The model under review builds one solid part; all positions refer to its coordinate system, in mm. A direction names the side the tool comes from. Coordinates: 2 decimals unless noted, no trailing zeros. Write each loop counter-clockwise with the first axis right and the second up, starting at its lowest first coordinate (ties: lowest second). Pieces come first, ordered by that corner, then holes.
1) Add section A-A, the plane z = -8.5. State the section outline as (x, y) points.
2) Machinability: for faces 1 (the flat face through (-1.65, -1.74, 3.77)), 2 (the cylindrical face through (-0.54, 2.44, -10.31)), which of the approach directions +Z, -Z, +X, -X, +Y, -Y give a long, thin tool a straight path to every point of the face, cutting with its end or side? Answer none if there is none.
3) For P1, Ø1, axis at y = -1, z = -2.5, coming from the -X side; P2, Ø1, axis at x = 1, y = 3.5, coming from the -Z side; P3, Ø0.9, axis at x = 1, y = -1.5, coming from the +Z side, all flat-tipped, find the tip position at first contact; note any pin that passes through.
4) For line 1 (Z direction, x = 3, y = -1); line 2 (Y direction, x = 0, z = -1.75); line 3 (X direction, y = 1.5, z = -19), list the stretches that pass through material, from the lowest coordinate up.
5) Mouldability with a two-part tool opening along X and no side actions: class faces 3 (the cylindrical face through (2.285, -3.584, 2.469)), 4 (the flat face through (1.65, 1.74, 3.77)), 5 (the flat face through (2, -2, 5)) as released by +X, released by -X, zero draft, split by the parting line, or undercut.
Solid Edge part; units mm, degrees
sketch "Sketch1" plane through (0, 0, 0) normal (0, -1, 0) x (1, 0, 0)
  line L0 (4.25, 5) -> (4.25, 0)
  line L1 (4.25, 0) -> (2.85, 0)
  line L2 (2.85, 0) -> (2.5, -0.6062)
  line L3 (2.5, -0.6062) -> (2.5, -20)
  line L4 (2.5, -20) -> (0, -20)
  line L5 (2.3, 2.5) -> (0, 1.1721)
  line L6 (2.3, 5) -> (2.3, 2.5)
  line L7 (4.25, 5) -> (2.3, 5)
revolve "RevolvedProtrusion1" add sketch "Sketch1" angle 360 about axis through (0, 0, -6) along (0, 0, 1)
cosmetic_thread "Thread1"
chamfer "Chamfer_1" distance 0.25 angle 45 1 edges at (-2.5, 0, -20)
fillet "Round_1" radius 0.3 2 edges at (-4.25, 0, 0) (-4.25, 0, 5)
sketch "Sketch2" plane through (0, 0, 5) normal (0, 0, 1) x (0, 1, 0)
  line L0 (-2.3, 1.3279) -> (-2.3, -1.3279)
  line L1 (0, -2.6558) -> (-2.3, -1.3279)
  line L2 (2.3, -1.3279) -> (0, -2.6558)
  line L3 (2.3, 1.3279) -> (2.3, -1.3279)
  line L4 (0, 2.6558) -> (2.3, 1.3279)
  line L5 (-2.3, 1.3279) -> (0, 2.6558)
extrude "Cutout1" cut sketch "Sketch2" against normal up to vertex (2.5 mm away)
properties material "Galvanized steel"
Geometry results:
1. outline: circle Ø5 at (0, 0)
2. face 1: +Z
2. face 2: -Z
3. P1: stops at x = -2.45
3. P2: stops at z = 0
3. P3: stops at z = 2.47
4. line 1: z = 0 to 5
4. line 2: y = -2.5 to 2.5
4. line 3: x = -2 to 2
5. face 3: split by the parting line
5. face 4: undercut
5. face 5: zero draft
